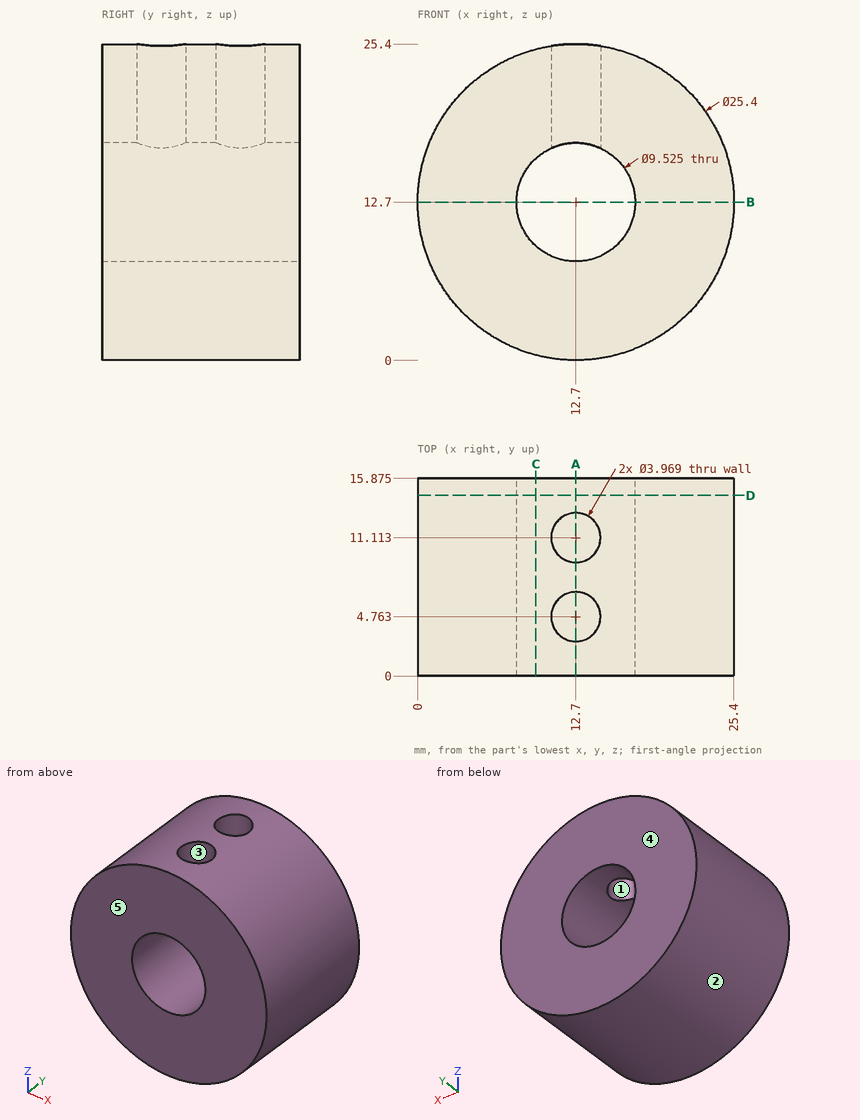
Study the drawing (mm; zero at the part's minimum x, y, z) and answer. A direction names the side the tool comes from. Give positions to 0.01 mm unless a question says otherwise; leave off trailing zeros. Loops run counter-clockwise (first coordinate to the right, second up) from the corner with the lowest first, then second, coordinate; pieces in that order, holes last. Notation, with made-up numbers: (-33.75, -40) - (-22.75, -40) arc R16 ccw to (-22.75, -27) - close; hole circle Ø10 at (-5.5, -16). An arc over 180 degrees is marked (long way). Return JSON: item names as keys, results as strings. Group by question number.
1. Find section C-C (x = 9.5). Write down the section's boundary in (y, z) (1 decimal), then the cut area to 3 significant figures.
2. Which of the six approach directions +Z, -Z, +X, -X, +Y, -Y give full straight-line access (tool end or side, diameter ignored) to the marked faces 1 and 2?
3. Determine the mould class of the marked faces 3, 4 and 5 for opening direction Y: pulls with the +Y half, pulls with the -Y half, needs draft (parallel to the pull), parting line crosses it, or undercut.
4. Find section B-B (z = 12.7). Write down the section's boundary in (x, y) (1 decimal).
5. Find section D-D (y = 14.5). Write down the section's boundary in (x, z) (1 decimal).
6. Straight lines are drawn through the part: line 1 (X direction, y = 9.25, z = 12.7); line 2 (X direction, y = 3, z = 16.5) (1 decimal); line 3 (Z direction, x = 15, y = 10.5). For each, find the intervals that lie inside material, in ascending order. Write a range as [from, to].
7. Given pin 1 Ø1 at (x, y) = (3.5, 6) entering from +Z; pin 2 Ø1 at (y, z) = (2.5, 18) entering from +X; pin 3 Ø1 at (y, z) = (14, 4.5) entering from -X, each flat-ended and moving along its own axis, determine where each tip first touches the part or whether it passes through.
8. Find section A-A (x = 12.7). Write down the section's boundary in (y, z) (1 decimal), then the cut area to 3 significant figures.
Verdict:
{
 "1": {"outline": "(0, 0.4) - (15.9, 0.4) - (15.9, 9.2) - (0, 9.2) - close; (0, 16.2) - (15.9, 16.2) - (15.9, 25) - (0, 25) - close", "area": "278 mm^2"},
 "2": {"face 1": "+Z", "face 2": "+Y, -Y"},
 "3": {"face 3": "undercut", "face 4": "pulls with the +Y half", "face 5": "pulls with the -Y half"},
 "4": {"outline": "(0, 0) - (7.9, 0) - (7.9, 15.9) - (0, 15.9) - close; (17.5, 0) - (25.4, 0) - (25.4, 15.9) - (17.5, 15.9) - close"},
 "5": {"outline": "circle Ø25.4 at (12.7, 12.7); hole circle Ø9.5 at (12.7, 12.7)"},
 "6": {"line 1": "x = [0, 7.94], [17.46, 25.4]", "line 2": "x = [0.6, 9.8], [15.6, 24.8]", "line 3": "z = [0.21, 8.53], [16.87, 25.19]"},
 "7": {"pin 1": "stops at z = 21.95", "pin 2": "stops at x = 24.46", "pin 3": "stops at x = 2.6"},
 "8": {"outline": "(0, 0) - (15.9, 0) - (15.9, 7.9) - (0, 7.9) - close; (0, 17.5) - (2.8, 17.5) - (2.8, 25.4) - (0, 25.4) - close; (6.7, 17.5) - (9.1, 17.5) - (9.1, 25.4) - (6.7, 25.4) - close; (13.1, 17.5) - (15.9, 17.5) - (15.9, 25.4) - (13.1, 25.4) - close", "area": "189 mm^2"}
}
